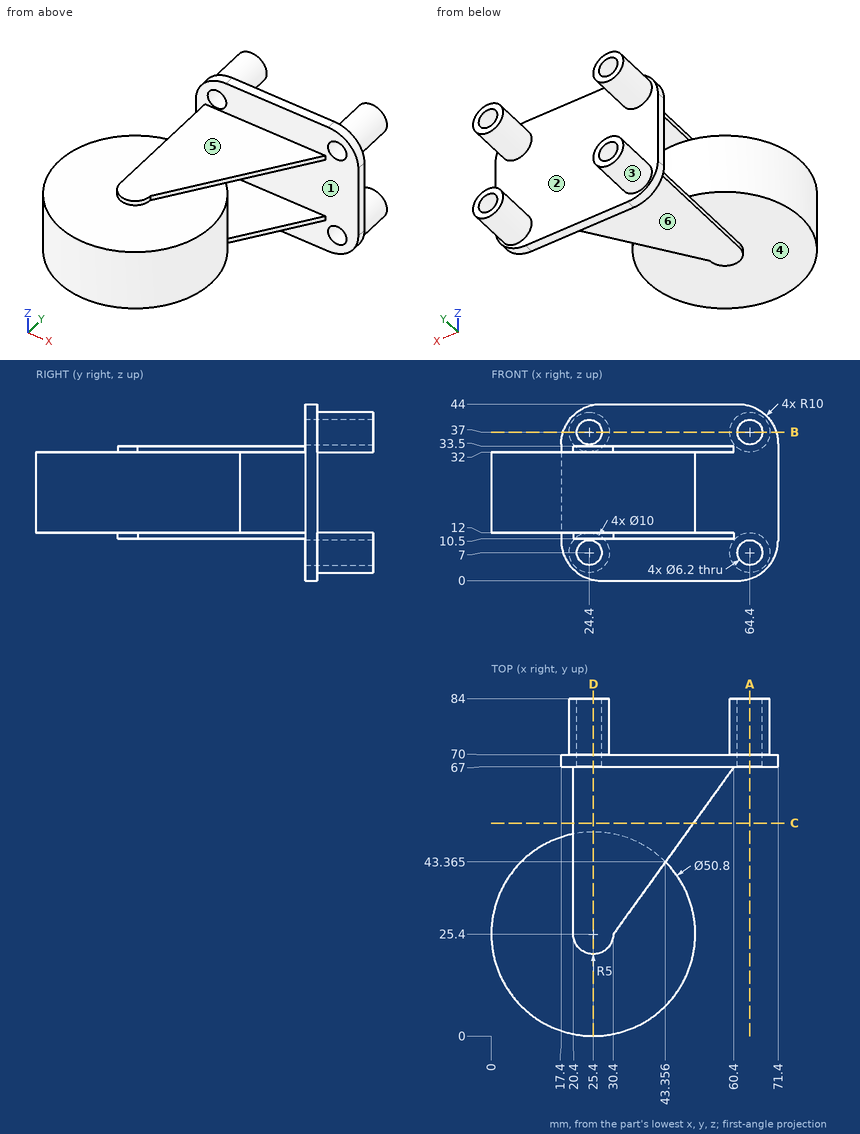
Job drawing, mm, ordinate dimensions from the low corner. One solid piece. A direction names the side the tool comes from. Round coordinates to 2 decimals unless told otherwise and drop trailing zeros. Loops run counter-clockwise (first coordinate to the right, second up) from the corner with the lowest first, then second, coordinate; pieces in that order, holes last. Notation, with made-up numbers: (57, -35.75) -> (105, -35.75) arc R6 ccw to (105, -24.75) -> close; hole circle Ø7 at (69, 50.25). An arc over 180 degrees is marked (long way). Use a Markdown table: item, result.
1) Cut at B-B, the plane z = 37. List the corners of the cut face in (x, y).
The answers:
| item | result |
|---|---|
| outline | (17.86, 67) -> (21.3, 67) -> (21.3, 84) -> (19.4, 84) -> (19.4, 70) -> (17.86, 70) -> close; (27.5, 67) -> (61.3, 67) -> (61.3, 84) -> (59.4, 84) -> (59.4, 70) -> (29.4, 70) -> (29.4, 84) -> (27.5, 84) -> close; (67.5, 67) -> (70.94, 67) -> (70.94, 70) -> (69.4, 70) -> (69.4, 84) -> (67.5, 84) -> close |
2) Drop flat-ended pins along their axis: pin 1 Ø6 at (x, y) = (19.5, 51.5) entering from +Z; pin 2 Ø12 at (x, y) = (34.5, 56.5) entering from -Z; pin 3 Ø1 at (y, z) = (69, 10.5) entering from -X; pin 4 Ø7 at (x, z) = (24.4, 7) entering from +Y. Give the stop position or say it passes through.
The answers:
| item | result |
|---|---|
| pin 1 | stops at z = 33.5 |
| pin 2 | stops at z = 10.5 |
| pin 3 | stops at x = 17.4 |
| pin 4 | stops at y = 84 |
3) Probe line 1 (X direction, y = 74.5, z = 7); line 2 (X direction, y = 79.5, z = 39); line 3 (Z direction, x = 64, y = 73). List the from-to ranges inside material, lowest first. Write a range as [from, to].
The answers:
| item | result |
|---|---|
| line 1 | x = [19.4, 21.3], [27.5, 29.4], [59.4, 61.3], [67.5, 69.4] |
| line 2 | x = [19.82, 22.03], [26.77, 28.98], [59.82, 62.03], [66.77, 68.98] |
| line 3 | z = [2.02, 3.93], [10.07, 11.98], [32.02, 33.93], [40.07, 41.98] |
4) Pull direction Y, two halves, no side cores. Call the marked faces 1, 2 and 3: pulls with the +Y half, pulls with the -Y half, needs draft (parallel to the pull), parting line crosses it, or undercut.
The answers:
| item | result |
|---|---|
| face 1 | undercut |
| face 2 | pulls with the +Y half |
| face 3 | needs draft |
5) Tool access for the marked faces 4, 5 and 6: list every direction of +Z, -Z, +X, -X, +Y, -Y with a clear straight run to the whole face (end or side of a thin tool).
The answers:
| item | result |
|---|---|
| face 4 | -Z, -Y |
| face 5 | +Z, +X, -X, -Y |
| face 6 | -Z, +X, -X, -Y |
6) Cut at C-C, the plane y = 53. List the corners of the cut face in (x, z).
The answers:
| item | result |
|---|---|
| outline | (20.4, 10.5) -> (50.3, 10.5) -> (50.3, 12) -> (20.4, 12) -> close; (20.4, 32) -> (50.3, 32) -> (50.3, 33.5) -> (20.4, 33.5) -> close |
7) Cut at A-A, the plane x = 64.4. List the corners of the cut face in (y, z).
The answers:
| item | result |
|---|---|
| outline | (67, 0.46) -> (70, 0.46) -> (70, 2) -> (84, 2) -> (84, 3.9) -> (67, 3.9) -> close; (67, 10.1) -> (84, 10.1) -> (84, 12) -> (70, 12) -> (70, 32) -> (84, 32) -> (84, 33.9) -> (67, 33.9) -> close; (67, 40.1) -> (84, 40.1) -> (84, 42) -> (70, 42) -> (70, 43.54) -> (67, 43.54) -> close |
8) Cut at D-D, the plane x = 25.4. State how many separate pieces and enclosed holes the cut face has, and give its area (3 significant figures).
The answers:
| item | result |
|---|---|
| separate pieces | 3 |
| enclosed holes | 1 |
| area | 1,360 mm2 |
